Could you check a few things on this model? Use its own coordinates, in mm. Give positions to 0.01 mm unless a question says otherwise; leave off trailing zeros. Order: outer loops, then holes, each group sorted by start corner. A loop starts at its lowest first (then second) coordinate and runs counter-clockwise, first axis right, second up. Notation, with made-up numbers: (46.25, 26.5) -> (76.25, 26.5) arc R15 ccw to (76.25, 54.5) -> close; hole circle Ø1 at (-2.5, 51). An arc over 180 degrees is marked (long way). One line per item, written item: value.
```python
from build123d import *

# Parameters (mm, degrees)
SKETCH1_R      = 1.7145
MAINBODY_DEPTH = 1.2
LARGEROUNDS_R  = 7.5184
SMALLROUNDS_R  = 1.5748


with BuildPart() as part:
    # Sketch1 → MainBody (new body)
    with BuildSketch(Plane.XY):
        Polygon((71.6788, -27.4828), (71.6788, 27.4828), (53.1114, 27.4828), (53.1114, 36.7792), (18.5674, 36.7792), (18.5674, 27.4828), (0, 27.4828), (0, -27.4828), (18.5674, -27.4828), (18.5674, -36.7792), (53.1114, -36.7792), (53.1114, -27.4828), align=None)
        with Locations((64.8462, -21.7424)):
            Circle(SKETCH1_R, mode=Mode.SUBTRACT)
        with Locations((6.8326, -21.7424)):
            Circle(SKETCH1_R, mode=Mode.SUBTRACT)
        with Locations((6.8326, 21.7424)):
            Circle(SKETCH1_R, mode=Mode.SUBTRACT)
        with Locations((64.8462, 21.7424)):
            Circle(SKETCH1_R, mode=Mode.SUBTRACT)
        with Locations((35.8394, -28.8671)):
            Circle(SKETCH1_R, mode=Mode.SUBTRACT)
        with Locations((35.8394, 28.8671)):
            Circle(SKETCH1_R, mode=Mode.SUBTRACT)
    extrude(amount=MAINBODY_DEPTH)

    # LargeRounds
    largerounds_edges = [part.edges().sort_by_distance(p)[0] for p in [
        (53.1114, -27.4828, 0.6),
        (18.5674, -27.4828, 0.6),
        (18.5674, 27.4828, 0.6),
        (53.1114, 27.4828, 0.6),
    ]]
    fillet(largerounds_edges, radius=LARGEROUNDS_R)

    # SmallRounds
    smallrounds_edges = [part.edges().sort_by_distance(p)[0] for p in [
        (53.1114, -36.7792, 0.6),
        (18.5674, -36.7792, 0.6),
        (0, -27.4828, 0.6),
        (0, 27.4828, 0.6),
        (18.5674, 36.7792, 0.6),
        (53.1114, 36.7792, 0.6),
        (71.6788, 27.4828, 0.6),
        (71.6788, -27.4828, 0.6),
    ]]
    fillet(smallrounds_edges, radius=SMALLROUNDS_R)


solid = part.part
```
1) If I drill on line 1 along X through (y, z) = (22, 0.6); line 2 along Y through (x, z) = (60.5, 1.05); line 3 along Y through (x, z) = (7.5, 0.35), over which ranges is the centre line in solid material (lowest first)?
Answer below:
line 1: x = 0 to 5.14, 8.53 to 63.15, 66.54 to 71.68
line 2: y = -27.48 to 27.48
line 3: y = -27.48 to -23.32, -20.16 to 20.16, 23.32 to 27.48
2) Suppose I cut it at C-C, the plane x = 67.5. Write out the boundary of the cut face in (y, z), then the cut area to 3 significant figures.
Answer below:
outline: (-27.48, 0) -> (27.48, 0) -> (27.48, 1.2) -> (-27.48, 1.2) -> close
area: 66.0 mm2
3) Suppose I cut it at A-A, the plane z = 0.7. State how many separate pieces and enclosed holes the cut face has, then the cut area to 3 significant figures.
Answer below:
separate pieces: 1
enclosed holes: 6
area: 4,570 mm2
4) Suppose I cut it at B-B, the plane x = 6. Write out the boundary of the cut face in (y, z).
Answer below:
outline: (-27.48, 0) -> (-23.24, 0) -> (-23.24, 1.2) -> (-27.48, 1.2) -> close; (-20.24, 0) -> (20.24, 0) -> (20.24, 1.2) -> (-20.24, 1.2) -> close; (23.24, 0) -> (27.48, 0) -> (27.48, 1.2) -> (23.24, 1.2) -> close
5) For P1, Ø2.5, axis at x = 64.85, y = 21.74, coming from the +Z side, with a flat end and sliding along its axis, tell me the tip position at first contact or that it passes through.
Answer below:
P1: passes through
6) We'd pull the mould along Y, two halves only. Please class faces 1 (the cylindrical face through (52.66, -36.31, 0.61)), 2 (the cylindrical face through (37.475, 29.382, 0.592)), 3 (the cylindrical face through (71.23, 27.01, 0.61)): +Y half, -Y half, draft (parallel to the pull), parting line (faces both ways), or undercut.
Answer below:
face 1: -Y half
face 2: undercut
face 3: +Y half
7) Suppose I cut it at D-D, the plane y = 31.5. Write out the boundary of the cut face in (x, z).
Answer below:
outline: (17.7, 0) -> (53.98, 0) -> (53.98, 1.2) -> (17.7, 1.2) -> close
